Source: CAD feature listing. Evaluate the final solid. Frame: model axes, mm. Face numbers are marked on the shaded views. A direction names the side the tool comes from. Round coordinates to 2 decimals unless told otherwise and drop trailing zeros. Order: outer loops, then holes, each group sorted by start corner. A loop starts at its lowest first (then second) coordinate and runs counter-clockwise, first axis right, second up. Notation, with made-up numbers: (21.25, 42.5) - (27.25, 42.5) arc R22 cw to (27.25, 59.5) - close; hole circle Ø9 at (6.25, 4.25). An arc over 180 degrees is marked (long way). Return JSON: item names as keys, results as strings. Group by question number.
1) Section D-D, the plane y = -14.5. Return loops of the section in (x, z).
2) Section A-A, the plane y = -57.5. Return loops of the section in (x, z), plus the area to 3 significant figures.
3) Ray query, line 1 (Z direction, x = 0, y = -40.5); line 2 (Z direction, x = 67, y = 3); line 3 (Y direction, x = 120, z = -36). Return the intervals inside material, ascending. Write a range as from..to.
4) Access query for the marked faces 3 and 4. Directions: +Z, -Z, +X, -X, +Y, -Y. A direction counts if a zero-diameter tool reaches every point of the face in a straight line with its end or side. Return the directions, or none.
5) Mould query, pull axis X, two halves, no side actions, for the marked faces 1 and 2. Classes: pulls with the +X half, pulls with the -X half, needs draft (parallel to the pull), parting line crosses it, or undercut.
6) Section C-C, the plane z = 23.5. Return loops of the section in (x, y).
7) Contact query for flat-ended pins moving along their axis: P1, Ø8, axis at y = -9.5, z = -10.5, coming from the -X side; P2, Ø5.5, axis at y = 18, z = -31, coming from the -X side; P3, Ø5.5, axis at y = 18.5, z = 32.5, coming from the -X side; P4, Ø18.5, axis at x = 250, z = 0, coming from the -Y side. Output: stop coordinate, or through.
8) Section B-B, the plane x = 64. Return loops of the section in (y, z), plus the area to 3 significant figures.
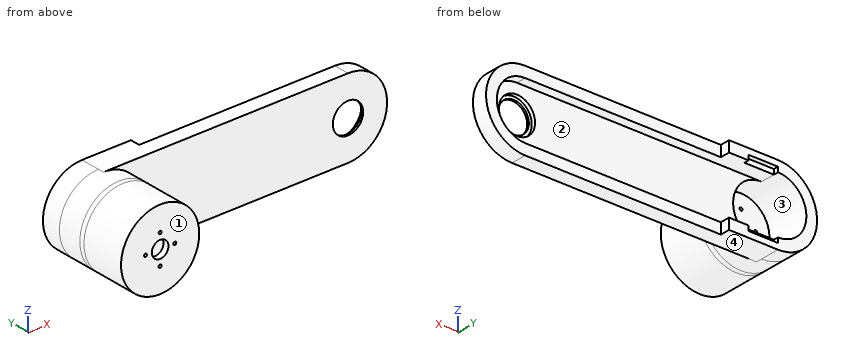
```python
from build123d import *

# Parameters (mm, degrees)
BOSS_EXTRUDE1_DEPTH     = 20
SKETCH2_R               = 40
SKETCH2_R_2             = 29
BOSS_EXTRUDE2_DEPTH     = 24.8
SKETCH3_R               = 40
BOSS_EXTRUDE3_DEPTH     = 5
BOSS_EXTRUDE4_DEPTH     = 6
SKETCH5_R               = 1.5
CUT_EXTRUDE1_DEPTH      = 45.8
CUT_EXTRUDE1_DEPTH_BACK = 6
SKETCH6_W               = 30
SKETCH6_H               = 5
CUT_EXTRUDE2_DEPTH      = 34
CUT_EXTRUDE2_DEPTH_BACK = 34
SKETCH7_R               = 18.5
SKETCH7_R_2             = 15.5
CUT_EXTRUDE3_DEPTH      = 4
SKETCH7_2_R             = 15.5
CUT_EXTRUDE4_DEPTH      = 21
CUT_EXTRUDE4_DEPTH_BACK = 30.8
CUT_EXTRUDE5_DEPTH      = 10
SKETCH10_R              = 40
SKETCH10_R_2            = 1.5
BOSS_EXTRUDE5_DEPTH     = 45
SKETCH11_R              = 8.5
CUT_EXTRUDE6_DEPTH      = 6


with BuildPart() as part:
    # Sketch1 → Boss-Extrude1 (new body)
    with BuildSketch(Plane(origin=(0, 0, 0), x_dir=(1, 0, 0), z_dir=(0, 1, 0))):
        with BuildLine():
            Line((0, -40), (250, -40))
            ThreePointArc((250, -40), (290, 0), (250, 40))
            Line((250, 40), (0, 40))
            ThreePointArc((0, 40), (-40, 0), (0, -40))
        make_face()
        with BuildLine():
            Line((0, 29), (250, 29))
            ThreePointArc((250, 29), (279, 0), (250, -29))
            Line((250, -29), (0, -29))
            ThreePointArc((0, -29), (-29, 0), (0, 29))
        make_face(mode=Mode.SUBTRACT)
    extrude(amount=BOSS_EXTRUDE1_DEPTH)

    # Sketch2 → Boss-Extrude2 (add)
    with BuildSketch(Plane.XZ):
        Circle(SKETCH2_R)
        Circle(SKETCH2_R_2, mode=Mode.SUBTRACT)
    extrude(amount=BOSS_EXTRUDE2_DEPTH)

    # Sketch3 → Boss-Extrude3 (add)
    with BuildSketch(Plane.XZ.offset(24.8)):
        Circle(SKETCH3_R)
    extrude(amount=BOSS_EXTRUDE3_DEPTH)

    # Sketch4 → Boss-Extrude4 (add)
    with BuildSketch(Plane.XZ):
        with BuildLine():
            Line((250, -40), (0, -40))
            ThreePointArc((0, -40), (14.832396974, -37.148351242), (27.549954628, -29))
            ThreePointArc((27.549954628, -29), (40, 0), (27.549954628, 29))
            ThreePointArc((27.549954628, 29), (14.832396974, 37.148351242), (0, 40))
            Line((0, 40), (250, 40))
            ThreePointArc((250, 40), (290, 0), (250, -40))
        make_face()
    extrude(amount=BOSS_EXTRUDE4_DEPTH)

    # Sketch5 → Cut-Extrude1 (cut, two sides)
    with BuildSketch(Plane(origin=(0, -24.8, 0), x_dir=(1, 0, 0), z_dir=(0, 1, 0))) as cut_extrude1_sk:
        with Locations((0, 15)):
            Circle(SKETCH5_R)
        with Locations((15, 0)):
            Circle(SKETCH5_R)
        with Locations((0, -15)):
            Circle(SKETCH5_R)
        with Locations((-15, 0)):
            Circle(SKETCH5_R)
    extrude(amount=CUT_EXTRUDE1_DEPTH, mode=Mode.SUBTRACT)
    extrude(cut_extrude1_sk.sketch, amount=-CUT_EXTRUDE1_DEPTH_BACK, mode=Mode.SUBTRACT)

    # Sketch6 → Cut-Extrude2 (cut, two sides)
    with BuildSketch(Plane.XY) as cut_extrude2_sk:
        with Locations((15, 17.5)):
            Rectangle(SKETCH6_W, SKETCH6_H)
    extrude(amount=CUT_EXTRUDE2_DEPTH, mode=Mode.SUBTRACT)
    extrude(cut_extrude2_sk.sketch, amount=-CUT_EXTRUDE2_DEPTH_BACK, mode=Mode.SUBTRACT)

    # Sketch7 → Cut-Extrude3 (cut)
    with BuildSketch(Plane(origin=(0, 0, 0), x_dir=(1, 0, 0), z_dir=(0, 1, 0))):
        with Locations((250, 0)):
            Circle(SKETCH7_R)
        with Locations((250, 0)):
            Circle(SKETCH7_R_2, mode=Mode.SUBTRACT)
    extrude(amount=-CUT_EXTRUDE3_DEPTH, mode=Mode.SUBTRACT)

    # Sketch7<2> → Cut-Extrude4 (cut, two sides)
    with BuildSketch(Plane(origin=(0, 0, 0), x_dir=(1, 0, 0), z_dir=(0, 1, 0))) as cut_extrude4_sk:
        with Locations((250, 0)):
            Circle(SKETCH7_2_R)
    extrude(amount=CUT_EXTRUDE4_DEPTH, mode=Mode.SUBTRACT)
    extrude(cut_extrude4_sk.sketch, amount=-CUT_EXTRUDE4_DEPTH_BACK, mode=Mode.SUBTRACT)

    # Sketch9 → Cut-Extrude5 (cut)
    with BuildSketch(Plane(origin=(0, 20, 0), x_dir=(1, 0, 0), z_dir=(0, 1, 0))):
        with BuildLine():
            Line((50, -40), (250, -40))
            ThreePointArc((250, -40), (290, 0), (250, 40))
            Line((250, 40), (50, 40))
            Line((50, 40), (50, -40))
        make_face()
    extrude(amount=-CUT_EXTRUDE5_DEPTH, mode=Mode.SUBTRACT)

    # Sketch10 → Boss-Extrude5 (add)
    with BuildSketch(Plane.XZ.offset(29.8)):
        Circle(SKETCH10_R)
        with Locations((-15, 0)):
            Circle(SKETCH10_R_2, mode=Mode.SUBTRACT)
        with Locations((0, -15)):
            Circle(SKETCH10_R_2, mode=Mode.SUBTRACT)
        with Locations((15, 0)):
            Circle(SKETCH10_R_2, mode=Mode.SUBTRACT)
        with Locations((0, 15)):
            Circle(SKETCH10_R_2, mode=Mode.SUBTRACT)
    extrude(amount=BOSS_EXTRUDE5_DEPTH)

    # Sketch11 → Cut-Extrude6 (cut)
    with BuildSketch(Plane.XZ.offset(74.8)):
        Circle(SKETCH11_R)
    extrude(amount=-CUT_EXTRUDE6_DEPTH, mode=Mode.SUBTRACT)


solid = part.part
```
Geometry check:
{
 "1": {"outline": "circle Ø80 at (0, 0); hole circle Ø58 at (0, 0)"},
 "2": {"outline": "circle Ø80 at (0, 0); hole circle Ø3 at (-15, 0); hole circle Ø3 at (0, -15); hole circle Ø3 at (0, 15); hole circle Ø3 at (15, 0)", "area": "5,000 mm2"},
 "3": {"line 1": "-40..-16.5, -13.5..13.5, 16.5..40", "line 2": "-40..-29, 29..40", "line 3": "-6..10"},
 "4": {"face 3": "+Y", "face 4": "-Z, +X, -X, +Y, -Y"},
 "5": {"face 1": "needs draft", "face 2": "undercut"},
 "6": {"outline": "(-32.37, -74.8) - (32.37, -74.8) - (32.37, -6) - (282.37, -6) - (282.37, 10) - (266.99, 10) - (266.99, 0) - (16.99, 0) - (16.99, -24.8) - (-16.99, -24.8) - (-16.99, 20) - (-32.37, 20) - close"},
 "7": {"P1": "x = -39.47", "P2": "x = -28.32", "P3": "x = -26.74", "P4": "through"},
 "8": {"outline": "(-6, -40) - (10, -40) - (10, -29) - (0, -29) - (0, 29) - (10, 29) - (10, 40) - (-6, 40) - close", "area": "700 mm2"}
}
